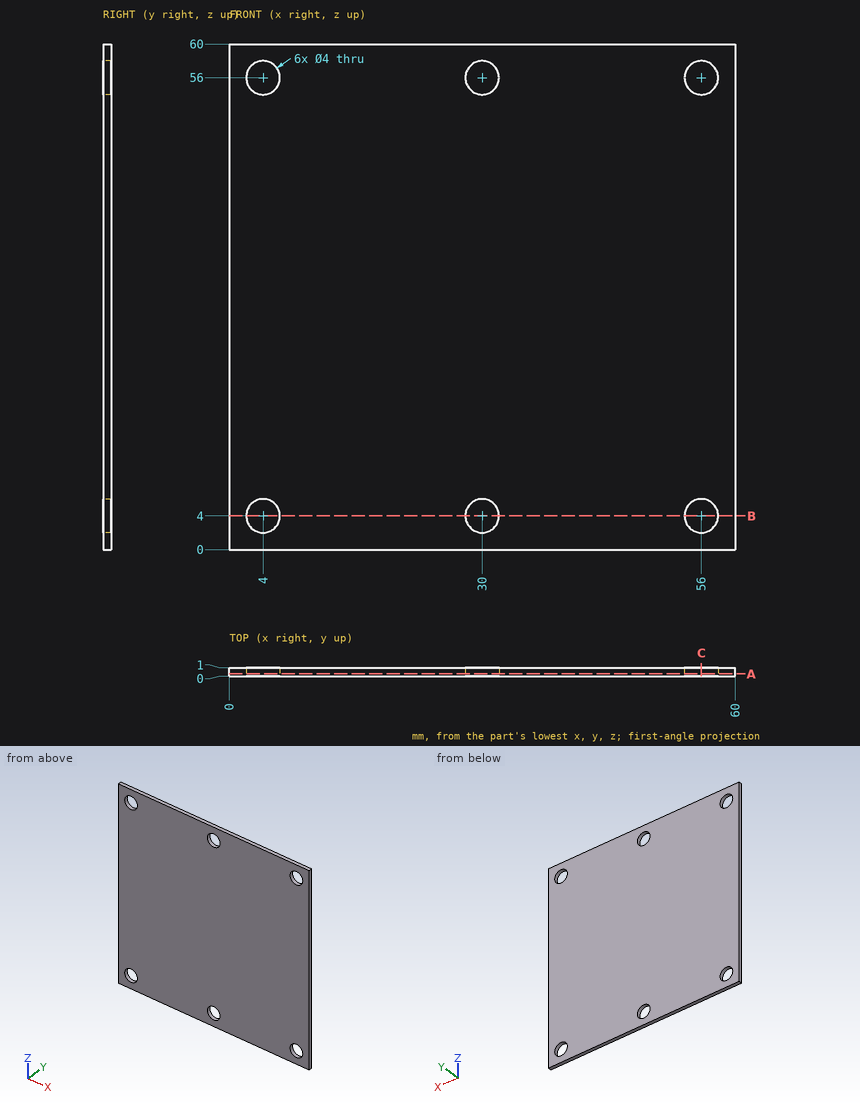
Study the drawing (mm; zero at the part's minimum x, y, z) and answer. Coordinates: 2 decimals unless noted, no trailing zeros. Write each loop counter-clockwise with the first axis right and the second up, starting at its lowest first coordinate (ties: lowest second). Pieces come first, ordered by that corner, then holes. Notation, with made-up numbers: (49.25, 48.5) - (108.25, 48.5) arc R13 cw to (108.25, 63.5) - close; hole circle Ø11 at (-32.5, 62.5). An arc over 180 degrees is marked (long way). Return JSON: item names as keys, results as strings. Group by question number.
1. A cutting plane is placed at C-C, the plane x = 56. Determine the outline of the cut face in (y, z).
2. Straight lines are drawn through the part: L1, parallel to Z at x = 30, y = 0.8; L2, parallel to X at y = 0.5, z = 4. For each, find the intervals that lie inside material, in ascending order.
3. A cutting plane is placed at B-B, the plane z = 4. Determine the outline of the cut face in (x, y), plus the area to 3 significant figures.
4. A cutting plane is placed at A-A, the plane y = 0.25. Determine the outline of the cut face in (x, z), plus the area to 3 significant figures.
5. Given pin 1 (2.5 mm diameter, centred on x = 30, z = 56, fed in from +Y), flat-ended and moving along its own axis, determine where the tip first touches the part or whether it passes through.
Ans:
{
 "1": {"outline": "(0, 0) - (1, 0) - (1, 2) - (0, 2) - close; (0, 6) - (1, 6) - (1, 54) - (0, 54) - close; (0, 58) - (1, 58) - (1, 60) - (0, 60) - close"},
 "2": {"L1": "0 to 2, 6 to 54, 58 to 60", "L2": "0 to 2, 6 to 28, 32 to 54, 58 to 60"},
 "3": {"outline": "(0, 0) - (2, 0) - (2, 1) - (0, 1) - close; (6, 0) - (28, 0) - (28, 1) - (6, 1) - close; (32, 0) - (54, 0) - (54, 1) - (32, 1) - close; (58, 0) - (60, 0) - (60, 1) - (58, 1) - close", "area": "48.0 mm²"},
 "4": {"outline": "(0, 0) - (60, 0) - (60, 60) - (0, 60) - close; hole circle Ø4 at (4, 4); hole circle Ø4 at (4, 56); hole circle Ø4 at (30, 4); hole circle Ø4 at (30, 56); hole circle Ø4 at (56, 4); hole circle Ø4 at (56, 56)", "area": "3,520 mm²"},
 "5": {"pin 1": "through"}
}
